Build history of the part. All positions in model axes, mm. A direction names the side the tool comes from. Give positions to 0.01 mm unless a question says otherwise; leave off trailing zeros. Write each loop counter-clockwise with the first axis right and the second up, starting at its lowest first coordinate (ties: lowest second). Pieces come first, ordered by that corner, then holes. Notation, with made-up numbers: (84.5, -32) -> (92.5, -32) arc R20 ccw to (92.5, -6) -> close; hole circle Ø11 at (23, 31.25). An arc over 180 degrees is marked (long way). Put each result on its own line as item: value.
from build123d import *

# Parameters (mm, degrees)
SKETCH1_R             = 30
BOSS_EXTRUDE1_DEPTH   = 50
SKETCH2_R             = 50
BOSS_EXTRUDE2_DEPTH   = 15
BOSS_EXTRUDE3_DEPTH   = 5
CUT_EXTRUDE1_DEPTH    = 196
F_1_0MM_DOWEL_HOLE1_D = 30


with BuildPart() as part:
    # Sketch1 → Boss-Extrude1 (new, symmetric)
    with BuildSketch(Plane.XY):
        Circle(SKETCH1_R)
    extrude(amount=BOSS_EXTRUDE1_DEPTH, both=True)



with BuildPart() as body_2:
    # Sketch2 → Boss-Extrude2 (new, symmetric)
    with BuildSketch(Plane.XY):
        with Locations((80, -80)):
            Circle(SKETCH2_R)
    extrude(amount=BOSS_EXTRUDE2_DEPTH, both=True)


with BuildPart() as part_1:
    add(part.part)

    add(body_2.part)  # Boss-Extrude3 merges body 2
    # Sketch3 → Boss-Extrude3 (add, symmetric)
    with BuildSketch(Plane.XY):
        Polygon((17.129116361, 24.629116361), (108.548527268, -38.951472732), (44.477364607, -115.187247331), (-30, -40), (-30, 0), align=None)
    extrude(amount=BOSS_EXTRUDE3_DEPTH, both=True)

    # Sketch4 → Cut-Extrude1 (cut, through all)
    with BuildSketch(Plane.XY.offset(15)):
        with BuildLine():
            Line((110, -80), (110, -155.272597881))
            ThreePointArc((110, -155.272597881), (80, -185.272597881), (50, -155.272597881))
            Line((50, -155.272597881), (50, -80))
            ThreePointArc((50, -80), (80, -50), (110, -80))
        make_face()
    extrude(amount=-CUT_EXTRUDE1_DEPTH, mode=Mode.SUBTRACT)

    # Ø1.0mm Dowel Hole1 (through all)
    with Locations(Plane.XY.offset(50)):
        with Locations((0, 0)):
            Hole(F_1_0MM_DOWEL_HOLE1_D / 2)


solid = part_1.part
1) Pull direction Y, two halves, no side cores. Call faces 1 (the flat face through (110, -100, 0)), 2 (the cylindrical face through (79.34, -50.007, 0.21)), 3 (the flat face through (62.199, -6.716, 0.07)), 4 (the cylindrical face through (14.985, 0.66, -0.7)): released by +Y, released by -Y, zero draft, split by the parting line, or undercut.
Filled sheet:
face 1: zero draft
face 2: released by -Y
face 3: released by +Y
face 4: undercut
2) Slice it at B-B (x = 0). Write the cut outline in (y, z), plus the area to 3 significant figures.
Filled sheet:
outline: (-70.29, -5) -> (-30, -5) -> (-30, -50) -> (-15, -50) -> (-15, 50) -> (-30, 50) -> (-30, 5) -> (-70.29, 5) -> close; (15, -50) -> (30, -50) -> (30, 50) -> (15, 50) -> close
area: 3,400 mm2
3) Slice it at C-C (y = -9). Write the cut outline in (x, z), plus the area to 3 significant figures.
Filled sheet:
outline: (-30, -5) -> (-28.62, -5) -> (-28.62, -50) -> (-12, -50) -> (-12, 50) -> (-28.62, 50) -> (-28.62, 5) -> (-30, 5) -> close; (12, -50) -> (28.62, -50) -> (28.62, -5) -> (65.48, -5) -> (65.48, 5) -> (28.62, 5) -> (28.62, 50) -> (12, 50) -> close
area: 3,710 mm2
4) Slice it at A-A (z = 2). Write the cut outline in (x, y).
Filled sheet:
outline: (-30, -40) -> (44.48, -115.19) arc R50 ccw to (50, -120) -> (50, -80) arc R30 cw to (110, -80) -> (110, -120) arc R50 ccw to (108.55, -38.95) -> (17.13, 24.63) arc R30 ccw to (-30, 0) -> close; hole circle Ø30 at (0, 0)
5) Pin check, flat tips, straight feed: pin 1 (12 mm diameter, centred on x = 67, z = -17, fed in from +Y); pin 2 (1.5 mm diameter, centred on y = -23.5, z = 19.5, fed in from +X); pin 3 (4 mm diameter, centred on x = 46.5, y = 1.5, fed in from -Z); pin 4 (12 mm diameter, centred on x = 33.5, y = 6, fed in from -Z). Stop position of each tip, or through.
Filled sheet:
pin 1: y = -30.54
pin 2: x = 19.56
pin 3: z = -5
pin 4: z = -50
6) Slice it at D-D (x = 52). Write the cut outline in (y, z), plus the area to 3 significant figures.
Filled sheet:
outline: (-69.23, -15) -> (-38.58, -15) -> (-38.58, -5) -> (0.38, -5) -> (0.38, 5) -> (-38.58, 5) -> (-38.58, 15) -> (-69.23, 15) -> close
area: 1,310 mm2
7) Tool access for faces 5 (the flat face through (24, -40, -5)), 6 (the cylindrical face through (-3.905, 29.745, 0.7)), 7 (the flat face through (24, -40, 5)), 8 (the flat face through (50, -100, 0)): list every direction of +Z, -Z, +X, -X, +Y, -Y with a clear straight run to the whole face (end or side of a thin tool).
Filled sheet:
face 5: -Z
face 6: none
face 7: +Z
face 8: +Z, -Z, -Y
8) Wall check: L1, parallel to Y at x = 0, z = -8.5; L2, parallel to Z at x = -16.5, y = -35; L3, parallel to Y at x = 0, z = 4. Give the ranges that are in metal, low to high.
Filled sheet:
L1: -30 to -15, 15 to 30
L2: -5 to 5
L3: -70.29 to -15, 15 to 30
